The listing builds one solid part. Answer for the finished solid, in the listing's coordinates (mm). Give positions to 0.01 mm unless a question says otherwise; leave off trailing zeros. Order: outer loops, then holes, each group sorted by start corner. A loop starts at its lowest first (then second) coordinate and runs counter-clockwise, first axis right, second up. Notation, with made-up numbers: (-23, -28.5) -> (14, -28.5) arc R22 cw to (14, -5.5) -> close; hole circle Ø8 at (-7.5, 84). An arc over 180 degrees is marked (long way). Answer as a JSON object with one key per item and string values. Group by question number.
```python
from build123d import *

# Parameters (mm, degrees)
SKETCH_3_W          = 4
SKETCH_3_H          = 120
EXTRUDE_2_DEPTH     = 2
SKETCH_4_R          = 5
EXTRUDE_3_DEPTH     = 4
SKETCH_9_R          = 5
EXTRUDE_7_DEPTH     = 4
EXTRUDE_7_2_DEPTH   = 4
EXTRUDE_8_DEPTH     = 2
SKETCH_5_R          = 2.5
CUT_EXTRUDE_3_DEPTH = 175.851401773
SKETCH_11_W         = 4
SKETCH_11_H         = 2
EXTRUDE_9_DEPTH     = 10
SKETCH_12_R         = 5
EXTRUDE_10_DEPTH    = 4
CUT_EXTRUDE_4_REACH = 135.503
SKETCH_13_R         = 2
RIB_2_REACH         = 179.747
SKETCH_15_WALL_W    = 366.224417408
SKETCH_15_WALL_H    = 2


with BuildPart() as part:
    # Sketch 3 → Extrude 2 (new body)
    with BuildSketch(Plane(origin=(0, 0, 0), x_dir=(1, 0, 0), z_dir=(0, 1, 0))):
        with Locations((0, 108)):
            Rectangle(SKETCH_3_W, SKETCH_3_H)
    extrude(amount=EXTRUDE_2_DEPTH)

    # Sketch 4 → Extrude 3 (add)
    with BuildSketch(Plane(origin=(0, 0, 0), x_dir=(1, 0, 0), z_dir=(0, 1, 0))):
        with Locations(Location((0, 52, 0), (0, 0, 113.578178478))):
            Circle(SKETCH_4_R)
        with Locations(Location((0, 102, 0), (0, 0, 66.421821522))):
            Circle(SKETCH_4_R)
        with Locations(Location((0, 152, 0), (0, 0, 66.421821522))):
            Circle(SKETCH_4_R)
    extrude(amount=EXTRUDE_3_DEPTH)



with BuildPart() as body_2:
    # Sketch 9 → Extrude 7 (new body)
    with BuildSketch(Plane(origin=(0, 0, 0), x_dir=(1, 0, 0), z_dir=(0, 1, 0))):
        with Locations(Location((-43.301270189, 77, 0), (0, 0, 270))):
            Circle(SKETCH_9_R)
    extrude(amount=EXTRUDE_7_DEPTH)


with BuildPart() as body_3:
    # Sketch 9 → Extrude 7 2 (new body)
    with BuildSketch(Plane(origin=(0, 0, 0), x_dir=(1, 0, 0), z_dir=(0, 1, 0))):
        with Locations(Location((43.301270189, 77, 0), (0, 0, 90))):
            Circle(SKETCH_9_R)
    extrude(amount=EXTRUDE_7_2_DEPTH)


with BuildPart() as part_1:
    add(part.part)

    add(body_2.part)  # Extrude 8 merges body 2

    add(body_3.part)  # Extrude 8 merges body 3
    # Sketch 10 → Extrude 8 (add)
    with BuildSketch(Plane(origin=(0, 0, 0), x_dir=(1, 0, 0), z_dir=(0, 1, 0))):
        Polygon((0, 104.309401077), (-47.301270189, 77), (0, 49.690598923), (47.301270189, 77), align=None)
        Polygon((0, 99.690598923), (-39.301270189, 77), (0, 54.309401077), (39.301270189, 77), align=None, mode=Mode.SUBTRACT)
    extrude(amount=EXTRUDE_8_DEPTH)

    # Sketch 5 → Cut-Extrude 3 (cut, through all)
    with BuildSketch(Plane(origin=(0, 0, 0), x_dir=(1, 0, 0), z_dir=(0, 1, 0))):
        with Locations(Location((0, 102, 0), (0, 0, 270))):
            Circle(SKETCH_5_R)
        with Locations(Location((0, 52, 0), (0, 0, 270))):
            Circle(SKETCH_5_R)
        with Locations(Location((0, 152, 0), (0, 0, 270))):
            Circle(SKETCH_5_R)
        with Locations(Location((-43.301270189, 77, 0), (0, 0, 270))):
            Circle(SKETCH_5_R)
        with Locations(Location((43.301270189, 77, 0), (0, 0, 270))):
            Circle(SKETCH_5_R)
    extrude(amount=CUT_EXTRUDE_3_DEPTH, mode=Mode.SUBTRACT)

    # Sketch 11 → Extrude 9 (add)
    with BuildSketch(Plane(origin=(0, 0, 0), x_dir=(1, 0, 0), z_dir=(0, 1, 0))):
        with Locations((0, 169)):
            Rectangle(SKETCH_11_W, SKETCH_11_H)
    extrude(amount=EXTRUDE_9_DEPTH)

    # Sketch 12 → Extrude 10 (add)
    with BuildSketch(Plane(origin=(0, 0, -170), x_dir=(-1, 0, 0), z_dir=(0, 0, -1))):
        with Locations((0, 14)):
            Circle(SKETCH_12_R)
    extrude(amount=-EXTRUDE_10_DEPTH)

    # Sketch 13 → Cut-Extrude 4 (cut, up to next)
    with BuildSketch(Plane(origin=(0, 0, -170), x_dir=(-1, 0, 0), z_dir=(0, 0, -1)), mode=Mode.PRIVATE) as cut_extrude_4_sk1:
        with Locations((0, 14)):
            Circle(SKETCH_13_R)
    cut_extrude_4_tool1 = extrude(cut_extrude_4_sk1.sketch, amount=-CUT_EXTRUDE_4_REACH, mode=Mode.PRIVATE) & part_1.part
    add(cut_extrude_4_tool1.solids().sort_by_distance((0, 14, -170))[0], mode=Mode.SUBTRACT)

    # Sketch 15 wall → Rib 2 (add, up to next)
    with BuildSketch(Plane(origin=(0, 5.650617497, -163.373503951), x_dir=(0, -0.707106781187, 0.707106781187), z_dir=(0, -0.707106781187, -0.707106781187)), mode=Mode.PRIVATE) as rib_2_sk1:
        Rectangle(SKETCH_15_WALL_W, SKETCH_15_WALL_H)
    rib_2_tool1 = extrude(rib_2_sk1.sketch, amount=RIB_2_REACH, mode=Mode.PRIVATE) - part_1.part
    add(rib_2_tool1.solids().sort_by_distance((0, 5.650617497, -163.373503951))[0])


solid = part_1.part
```
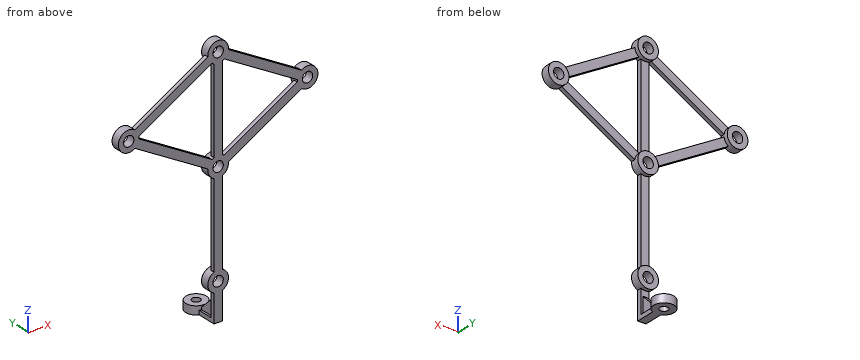
(1) Flat-ended cylindrical pins translate along their axes: pin 1 Ø3 at (x, z) = (1.5, -152) entering from +Y; pin 2 Ø12 at (x, z) = (27.5, -61) entering from -Y; pin 3 Ø12 at (x, z) = (-15.5, -69.5) entering from +Y; pin 4 Ø0.8 at (x, y) = (-1.5, 4) entering from +Z. Find the tip coordinate at first contact, or state that the pin passes through.
(2) Find the intervals of material crossed by line 1 along X through (y, z) = (2.35, -77); line 2 along X through (y, z) = (1.95, -77); line 3 along Z through (x, y) = (0, 0.85), in increasing order. Write a range as [from, to].
(3) A cutting plane is placed at D-D (y = 17.5). Determine the outline of the cut face in (x, z), and give its area (3 significant figures).
(4) A cutting plane is placed at C-C (z = -119.5). Determine the outline of the cut face in (x, y), and give its area (3 significant figures).
(5) A cutting plane is placed at B-B (x = -14.5). Determine the outline of the cut face in (y, z), and give its area (3 significant figures).
(6) A cutting plane is placed at A-A (z = -152). Determine the outline of the cut face in (x, y).
Check sheet entries:
{
 "1": {"pin 1": "stops at y = 4", "pin 2": "stops at y = 0", "pin 3": "stops at y = 2", "pin 4": "stops at z = -47.12"},
 "2": {"line 1": "x = [-48.3, -45.8], [-40.8, -38.3], [38.3, 40.8], [45.8, 48.3]", "line 2": "x = [-48.3, -45.8], [-40.8, -38.3], [-2, 2], [38.3, 40.8], [45.8, 48.3]", "line 3": "z = [-170, -154.5], [-149.5, -104.5], [-99.5, -54.5], [-49.5, -47]"},
 "3": {"outline": "(-3.57, -170) -> (3.57, -170) -> (3.57, -166) -> (-3.57, -166) -> close", "area": "28.6 mm2"},
 "4": {"outline": "(-2, 0) -> (2, 0) -> (2, 2) -> (-2, 2) -> close", "area": "8.00 mm2"},
 "5": {"outline": "(0, -95.94) -> (2, -95.94) -> (2, -91.32) -> (0, -91.32) -> close; (0, -62.68) -> (2, -62.68) -> (2, -58.06) -> (0, -58.06) -> close", "area": "18.5 mm2"},
 "6": {"outline": "(-5, 0) -> (-2.5, 0) -> (-2.5, 4) -> (-5, 4) -> close; (2.5, 0) -> (5, 0) -> (5, 4) -> (2.5, 4) -> close"}
}
